```python
from build123d import *

# Parameters (mm, degrees)
ESQUISSE1_W             = 165
ESQUISSE1_H             = 140
BOSS_EXTRU_1_DEPTH      = 12
ESQUISSE2_W             = 72
ESQUISSE2_H             = 65
ENL_V_MAT_EXTRU_1_DEPTH = 4.5
ENL_V_MAT_EXTRU_2_REACH = 218.723
ESQUISSE3_R             = 2.5
ESQUISSE4_R             = 4.5
ENL_V_MAT_EXTRU_3_DEPTH = 5
ESQUISSE5_W             = 165
ESQUISSE5_H             = 12
BOSS_EXTRU_2_DEPTH      = 45
ENL_V_MAT_EXTRU_4_REACH = 218.521
ESQUISSE6_R             = 5


with BuildPart() as part:
    # Esquisse1 → Boss.-Extru.1 (new body)
    with BuildSketch(Plane.XY):
        with Locations((82.5, 70)):
            Rectangle(ESQUISSE1_W, ESQUISSE1_H)
    extrude(amount=BOSS_EXTRU_1_DEPTH)

    # Esquisse2 → Enlèv. mat.-Extru.1 (cut)
    with BuildSketch(Plane(origin=(0, 0, 0), x_dir=(-1, 0, 0), z_dir=(0, 0, -1))):
        with Locations((-82.5, 70.5)):
            Rectangle(ESQUISSE2_W, ESQUISSE2_H)
    extrude(amount=-ENL_V_MAT_EXTRU_1_DEPTH, mode=Mode.SUBTRACT)

    # Esquisse3 → Enlèv. mat.-Extru.2 (cut, up to next)
    with BuildSketch(Plane.XY.offset(12), mode=Mode.PRIVATE) as enl_v_mat_extru_2_sk1:
        with Locations((158.5, 6.5)):
            Circle(ESQUISSE3_R)
    enl_v_mat_extru_2_tool1 = extrude(enl_v_mat_extru_2_sk1.sketch, amount=-ENL_V_MAT_EXTRU_2_REACH, mode=Mode.PRIVATE) & part.part
    # Esquisse3 → Enlèv. mat.-Extru.2 (cut, up to next)
    with BuildSketch(Plane.XY.offset(12), mode=Mode.PRIVATE) as enl_v_mat_extru_2_sk2:
        with Locations((158.5, 131.5)):
            Circle(ESQUISSE3_R)
    enl_v_mat_extru_2_tool2 = extrude(enl_v_mat_extru_2_sk2.sketch, amount=-ENL_V_MAT_EXTRU_2_REACH, mode=Mode.PRIVATE) & part.part
    # Esquisse3 → Enlèv. mat.-Extru.2 (cut, up to next)
    with BuildSketch(Plane.XY.offset(12), mode=Mode.PRIVATE) as enl_v_mat_extru_2_sk3:
        with Locations((126.5, 6.5)):
            Circle(ESQUISSE3_R)
    enl_v_mat_extru_2_tool3 = extrude(enl_v_mat_extru_2_sk3.sketch, amount=-ENL_V_MAT_EXTRU_2_REACH, mode=Mode.PRIVATE) & part.part
    # Esquisse3 → Enlèv. mat.-Extru.2 (cut, up to next)
    with BuildSketch(Plane.XY.offset(12), mode=Mode.PRIVATE) as enl_v_mat_extru_2_sk4:
        with Locations((126.5, 36.5)):
            Circle(ESQUISSE3_R)
    enl_v_mat_extru_2_tool4 = extrude(enl_v_mat_extru_2_sk4.sketch, amount=-ENL_V_MAT_EXTRU_2_REACH, mode=Mode.PRIVATE) & part.part
    # Esquisse3 → Enlèv. mat.-Extru.2 (cut, up to next)
    with BuildSketch(Plane.XY.offset(12), mode=Mode.PRIVATE) as enl_v_mat_extru_2_sk5:
        with Locations((158.5, 36.5)):
            Circle(ESQUISSE3_R)
    enl_v_mat_extru_2_tool5 = extrude(enl_v_mat_extru_2_sk5.sketch, amount=-ENL_V_MAT_EXTRU_2_REACH, mode=Mode.PRIVATE) & part.part
    # Esquisse3 → Enlèv. mat.-Extru.2 (cut, up to next)
    with BuildSketch(Plane.XY.offset(12), mode=Mode.PRIVATE) as enl_v_mat_extru_2_sk6:
        with Locations((126.5, 131.5)):
            Circle(ESQUISSE3_R)
    enl_v_mat_extru_2_tool6 = extrude(enl_v_mat_extru_2_sk6.sketch, amount=-ENL_V_MAT_EXTRU_2_REACH, mode=Mode.PRIVATE) & part.part
    # Esquisse3 → Enlèv. mat.-Extru.2 (cut, up to next)
    with BuildSketch(Plane.XY.offset(12), mode=Mode.PRIVATE) as enl_v_mat_extru_2_sk7:
        with Locations((126.5, 101.5)):
            Circle(ESQUISSE3_R)
    enl_v_mat_extru_2_tool7 = extrude(enl_v_mat_extru_2_sk7.sketch, amount=-ENL_V_MAT_EXTRU_2_REACH, mode=Mode.PRIVATE) & part.part
    # Esquisse3 → Enlèv. mat.-Extru.2 (cut, up to next)
    with BuildSketch(Plane.XY.offset(12), mode=Mode.PRIVATE) as enl_v_mat_extru_2_sk8:
        with Locations((158.5, 101.5)):
            Circle(ESQUISSE3_R)
    enl_v_mat_extru_2_tool8 = extrude(enl_v_mat_extru_2_sk8.sketch, amount=-ENL_V_MAT_EXTRU_2_REACH, mode=Mode.PRIVATE) & part.part
    # Esquisse3 → Enlèv. mat.-Extru.2 (cut, up to next)
    with BuildSketch(Plane.XY.offset(12), mode=Mode.PRIVATE) as enl_v_mat_extru_2_sk9:
        with Locations(Location((6.5, 6.5, 0), (0, 0, 180))):
            Circle(ESQUISSE3_R)
    enl_v_mat_extru_2_tool9 = extrude(enl_v_mat_extru_2_sk9.sketch, amount=-ENL_V_MAT_EXTRU_2_REACH, mode=Mode.PRIVATE) & part.part
    # Esquisse3 → Enlèv. mat.-Extru.2 (cut, up to next)
    with BuildSketch(Plane.XY.offset(12), mode=Mode.PRIVATE) as enl_v_mat_extru_2_sk10:
        with Locations(Location((6.5, 36.5, 0), (0, 0, 180))):
            Circle(ESQUISSE3_R)
    enl_v_mat_extru_2_tool10 = extrude(enl_v_mat_extru_2_sk10.sketch, amount=-ENL_V_MAT_EXTRU_2_REACH, mode=Mode.PRIVATE) & part.part
    # Esquisse3 → Enlèv. mat.-Extru.2 (cut, up to next)
    with BuildSketch(Plane.XY.offset(12), mode=Mode.PRIVATE) as enl_v_mat_extru_2_sk11:
        with Locations(Location((38.5, 6.5, 0), (0, 0, 180))):
            Circle(ESQUISSE3_R)
    enl_v_mat_extru_2_tool11 = extrude(enl_v_mat_extru_2_sk11.sketch, amount=-ENL_V_MAT_EXTRU_2_REACH, mode=Mode.PRIVATE) & part.part
    # Esquisse3 → Enlèv. mat.-Extru.2 (cut, up to next)
    with BuildSketch(Plane.XY.offset(12), mode=Mode.PRIVATE) as enl_v_mat_extru_2_sk12:
        with Locations(Location((38.5, 36.5, 0), (0, 0, 180))):
            Circle(ESQUISSE3_R)
    enl_v_mat_extru_2_tool12 = extrude(enl_v_mat_extru_2_sk12.sketch, amount=-ENL_V_MAT_EXTRU_2_REACH, mode=Mode.PRIVATE) & part.part
    # Esquisse3 → Enlèv. mat.-Extru.2 (cut, up to next)
    with BuildSketch(Plane.XY.offset(12), mode=Mode.PRIVATE) as enl_v_mat_extru_2_sk13:
        with Locations(Location((6.5, 101.5, 0), (0, 0, 180))):
            Circle(ESQUISSE3_R)
    enl_v_mat_extru_2_tool13 = extrude(enl_v_mat_extru_2_sk13.sketch, amount=-ENL_V_MAT_EXTRU_2_REACH, mode=Mode.PRIVATE) & part.part
    # Esquisse3 → Enlèv. mat.-Extru.2 (cut, up to next)
    with BuildSketch(Plane.XY.offset(12), mode=Mode.PRIVATE) as enl_v_mat_extru_2_sk14:
        with Locations(Location((38.5, 101.5, 0), (0, 0, 180))):
            Circle(ESQUISSE3_R)
    enl_v_mat_extru_2_tool14 = extrude(enl_v_mat_extru_2_sk14.sketch, amount=-ENL_V_MAT_EXTRU_2_REACH, mode=Mode.PRIVATE) & part.part
    # Esquisse3 → Enlèv. mat.-Extru.2 (cut, up to next)
    with BuildSketch(Plane.XY.offset(12), mode=Mode.PRIVATE) as enl_v_mat_extru_2_sk15:
        with Locations(Location((38.5, 131.5, 0), (0, 0, 180))):
            Circle(ESQUISSE3_R)
    enl_v_mat_extru_2_tool15 = extrude(enl_v_mat_extru_2_sk15.sketch, amount=-ENL_V_MAT_EXTRU_2_REACH, mode=Mode.PRIVATE) & part.part
    # Esquisse3 → Enlèv. mat.-Extru.2 (cut, up to next)
    with BuildSketch(Plane.XY.offset(12), mode=Mode.PRIVATE) as enl_v_mat_extru_2_sk16:
        with Locations(Location((6.5, 131.5, 0), (0, 0, 180))):
            Circle(ESQUISSE3_R)
    enl_v_mat_extru_2_tool16 = extrude(enl_v_mat_extru_2_sk16.sketch, amount=-ENL_V_MAT_EXTRU_2_REACH, mode=Mode.PRIVATE) & part.part
    add(enl_v_mat_extru_2_tool1.solids().sort_by_distance((158.5, 6.5, 12))[0], mode=Mode.SUBTRACT)
    add(enl_v_mat_extru_2_tool2.solids().sort_by_distance((158.5, 131.5, 12))[0], mode=Mode.SUBTRACT)
    add(enl_v_mat_extru_2_tool3.solids().sort_by_distance((126.5, 6.5, 12))[0], mode=Mode.SUBTRACT)
    add(enl_v_mat_extru_2_tool4.solids().sort_by_distance((126.5, 36.5, 12))[0], mode=Mode.SUBTRACT)
    add(enl_v_mat_extru_2_tool5.solids().sort_by_distance((158.5, 36.5, 12))[0], mode=Mode.SUBTRACT)
    add(enl_v_mat_extru_2_tool6.solids().sort_by_distance((126.5, 131.5, 12))[0], mode=Mode.SUBTRACT)
    add(enl_v_mat_extru_2_tool7.solids().sort_by_distance((126.5, 101.5, 12))[0], mode=Mode.SUBTRACT)
    add(enl_v_mat_extru_2_tool8.solids().sort_by_distance((158.5, 101.5, 12))[0], mode=Mode.SUBTRACT)
    add(enl_v_mat_extru_2_tool9.solids().sort_by_distance((6.5, 6.5, 12))[0], mode=Mode.SUBTRACT)
    add(enl_v_mat_extru_2_tool10.solids().sort_by_distance((6.5, 36.5, 12))[0], mode=Mode.SUBTRACT)
    add(enl_v_mat_extru_2_tool11.solids().sort_by_distance((38.5, 6.5, 12))[0], mode=Mode.SUBTRACT)
    add(enl_v_mat_extru_2_tool12.solids().sort_by_distance((38.5, 36.5, 12))[0], mode=Mode.SUBTRACT)
    add(enl_v_mat_extru_2_tool13.solids().sort_by_distance((6.5, 101.5, 12))[0], mode=Mode.SUBTRACT)
    add(enl_v_mat_extru_2_tool14.solids().sort_by_distance((38.5, 101.5, 12))[0], mode=Mode.SUBTRACT)
    add(enl_v_mat_extru_2_tool15.solids().sort_by_distance((38.5, 131.5, 12))[0], mode=Mode.SUBTRACT)
    add(enl_v_mat_extru_2_tool16.solids().sort_by_distance((6.5, 131.5, 12))[0], mode=Mode.SUBTRACT)

    # Esquisse4 → Enlèv. mat.-Extru.3 (cut)
    with BuildSketch(Plane.XY.offset(12)):
        with Locations((6.5, 131.5)):
            Circle(ESQUISSE4_R)
        with Locations((6.5, 101.5)):
            Circle(ESQUISSE4_R)
        with Locations((6.5, 36.5)):
            Circle(ESQUISSE4_R)
        with Locations((6.5, 6.5)):
            Circle(ESQUISSE4_R)
        with Locations((38.5, 6.5)):
            Circle(ESQUISSE4_R)
        with Locations((38.5, 36.5)):
            Circle(ESQUISSE4_R)
        with Locations((38.5, 101.5)):
            Circle(ESQUISSE4_R)
        with Locations((38.5, 131.5)):
            Circle(ESQUISSE4_R)
        with Locations(Location((158.5, 101.5, 0), (0, 0, 180))):
            Circle(ESQUISSE4_R)
        with Locations(Location((158.5, 131.5, 0), (0, 0, 180))):
            Circle(ESQUISSE4_R)
        with Locations(Location((126.5, 131.5, 0), (0, 0, 180))):
            Circle(ESQUISSE4_R)
        with Locations(Location((126.5, 101.5, 0), (0, 0, 180))):
            Circle(ESQUISSE4_R)
        with Locations(Location((126.5, 6.5, 0), (0, 0, 180))):
            Circle(ESQUISSE4_R)
        with Locations(Location((158.5, 6.5, 0), (0, 0, 180))):
            Circle(ESQUISSE4_R)
        with Locations(Location((158.5, 36.5, 0), (0, 0, 180))):
            Circle(ESQUISSE4_R)
        with Locations(Location((126.5, 36.5, 0), (0, 0, 180))):
            Circle(ESQUISSE4_R)
    extrude(amount=-ENL_V_MAT_EXTRU_3_DEPTH, mode=Mode.SUBTRACT)

    # Esquisse5 → Boss.-Extru.2 (add)
    with BuildSketch(Plane.XZ):
        with Locations((82.5, 6)):
            Rectangle(ESQUISSE5_W, ESQUISSE5_H)
    extrude(amount=BOSS_EXTRU_2_DEPTH)

    # Esquisse6 → Enlèv. mat.-Extru.4 (cut, up to next)
    with BuildSketch(Plane(origin=(0, 0, 4.5), x_dir=(-1, 0, 0), z_dir=(0, 0, -1)), mode=Mode.PRIVATE) as enl_v_mat_extru_4_sk1:
        with Locations((-57.5, 49)):
            Circle(ESQUISSE6_R)
    enl_v_mat_extru_4_tool1 = extrude(enl_v_mat_extru_4_sk1.sketch, amount=-ENL_V_MAT_EXTRU_4_REACH, mode=Mode.PRIVATE) & part.part
    # Esquisse6 → Enlèv. mat.-Extru.4 (cut, up to next)
    with BuildSketch(Plane(origin=(0, 0, 4.5), x_dir=(-1, 0, 0), z_dir=(0, 0, -1)), mode=Mode.PRIVATE) as enl_v_mat_extru_4_sk2:
        with Locations((-57.5, 69)):
            Circle(ESQUISSE6_R)
    enl_v_mat_extru_4_tool2 = extrude(enl_v_mat_extru_4_sk2.sketch, amount=-ENL_V_MAT_EXTRU_4_REACH, mode=Mode.PRIVATE) & part.part
    # Esquisse6 → Enlèv. mat.-Extru.4 (cut, up to next)
    with BuildSketch(Plane(origin=(0, 0, 4.5), x_dir=(-1, 0, 0), z_dir=(0, 0, -1)), mode=Mode.PRIVATE) as enl_v_mat_extru_4_sk3:
        with Locations((-107.5, 49)):
            Circle(ESQUISSE6_R)
    enl_v_mat_extru_4_tool3 = extrude(enl_v_mat_extru_4_sk3.sketch, amount=-ENL_V_MAT_EXTRU_4_REACH, mode=Mode.PRIVATE) & part.part
    # Esquisse6 → Enlèv. mat.-Extru.4 (cut, up to next)
    with BuildSketch(Plane(origin=(0, 0, 4.5), x_dir=(-1, 0, 0), z_dir=(0, 0, -1)), mode=Mode.PRIVATE) as enl_v_mat_extru_4_sk4:
        with Locations((-107.5, 69)):
            Circle(ESQUISSE6_R)
    enl_v_mat_extru_4_tool4 = extrude(enl_v_mat_extru_4_sk4.sketch, amount=-ENL_V_MAT_EXTRU_4_REACH, mode=Mode.PRIVATE) & part.part
    add(enl_v_mat_extru_4_tool1.solids().sort_by_distance((57.5, 49, 4.5))[0], mode=Mode.SUBTRACT)
    add(enl_v_mat_extru_4_tool2.solids().sort_by_distance((57.5, 69, 4.5))[0], mode=Mode.SUBTRACT)
    add(enl_v_mat_extru_4_tool3.solids().sort_by_distance((107.5, 49, 4.5))[0], mode=Mode.SUBTRACT)
    add(enl_v_mat_extru_4_tool4.solids().sort_by_distance((107.5, 69, 4.5))[0], mode=Mode.SUBTRACT)


solid = part.part
```
Check sheet for the modelled part. Datum: model origin and axes. Units: mm. A direction names the side the tool comes from. Coordinates: 2 decimals unless noted, no trailing zeros. Write each loop counter-clockwise with the first axis right and the second up, starting at its lowest first coordinate (ties: lowest second). Pieces come first, ordered by that corner, then holes. Notation, with made-up numbers: (11, 85) -> (57, 85) arc R31 cw to (57, 116) -> close; hole circle Ø1 at (63, -12). An arc over 180 degrees is marked (long way). Use a Markdown table: item, result.
1. Sectioned sample at C-C (x = 38.5). Give the number of separate pieces and of enclosed holes in the cut face, plus the area to 3 significant figures.
Reported:
| item | result |
|---|---|
| separate pieces | 5 |
| enclosed holes | 0 |
| area | 1,900 mm2 |
2. Scan lines: line 1 along Y through (x, z) = (6.5, 2.75); line 2 along Y through (x, z) = (158.5, 8.1); line 3 along X through (y, z) = (131.5, 4.25). Record each from-to range of solid material in increasing order.
Reported:
| item | result |
|---|---|
| line 1 | y = -45 to 4, 9 to 34, 39 to 99, 104 to 129, 134 to 140 |
| line 2 | y = -45 to 2, 11 to 32, 41 to 97, 106 to 127, 136 to 140 |
| line 3 | x = 0 to 4, 9 to 36, 41 to 124, 129 to 156, 161 to 165 |
3. Release check for a two-part mould opening along X. For faces 1 (the flat face through (40.4, 4.6, 7)), 2 (the cylindrical face through (61.185, 72.379, 8.198)) record: pulls with the +X half, pulls with the -X half, needs draft (parallel to the pull), parting line crosses it, or undercut.
Reported:
| item | result |
|---|---|
| face 1 | undercut |
| face 2 | undercut |
4. Tool access check on faces 3 (the cylindrical face through (160.885, 102.251, 3.549)), 4 (the flat face through (40.4, 34.6, 7)), 5 (the flat face through (83, 71, 4.5)). Record the directions out of +Z, -Z, +X, -X, +Y, -Y that give a thin tool (end or side, any length) a straight path to the whole face; none if there is none.
Reported:
| item | result |
|---|---|
| face 3 | +Z, -Z |
| face 4 | +Z |
| face 5 | -Z |
5. Sectioned sample at A-A (x = 107.5). Enter the section's corners in (y, z), plus the area to 3 significant figures.
Reported:
| item | result |
|---|---|
| outline | (-45, 0) -> (38, 0) -> (38, 4.5) -> (44, 4.5) -> (44, 12) -> (-45, 12) -> close; (54, 4.5) -> (64, 4.5) -> (64, 12) -> (54, 12) -> close; (74, 4.5) -> (103, 4.5) -> (103, 0) -> (140, 0) -> (140, 12) -> (74, 12) -> close |
| area | 1,780 mm2 |
6. Sectioned sample at B-B (y = 61.5). Enter the section's corners in (x, z).
Reported:
| item | result |
|---|---|
| outline | (0, 0) -> (46.5, 0) -> (46.5, 4.5) -> (118.5, 4.5) -> (118.5, 0) -> (165, 0) -> (165, 12) -> (0, 12) -> close |
